Check sheet for the modelled part. Datum: model origin and axes. Units: mm. A direction names the side the tool comes from. Give positions to 0.01 mm unless a question says otherwise; leave off trailing zeros. Order: outer loops, then holes, each group sorted by start corner. A loop starts at its lowest first (then second) coordinate and runs counter-clockwise, first axis right, second up.
Autodesk Fusion 360 part; units mm, degrees
sketch "スケッチ1" plane through (0, 0, 0) normal (0, 0, 1) x (1, 0, 0)
  line L0 (0, 0) -> (20, 0)
  line L1 (20, 0) -> (20, 20)
  line L2 (20, 20) -> (0, 20)
  line L3 (0, 20) -> (0, 0)
  dimension "d1" = 20
  dimension "d2" = 20
extrude "押し出し1" add sketch "スケッチ1" along normal blind 21
sketch "スケッチ2" plane through (20, 0, 0) normal (1, 0, 0) x (0, 1, 0)
  line L0 (0, 0) -> (20, 0)
  line L1 (20, 0) -> (20, 21)
  line L2 (20, 21) -> (0, 21)
  line L3 (0, 21) -> (0, 0)
  circle A0 centre (5, 5) radius 1.15
  dimension "d5" = 2.3
  dimension "d8" = 5
  dimension "d11" = 5
extrude "押し出し2" cut sketch "スケッチ2" against normal blind 25 contours A0
sketch "スケッチ7" plane through (0, 0, 21) normal (0, 0, 1) x (-1, 0, 0)
  line L0 (0, -20) -> (0, 0)
  line L1 (0, 0) -> (-20, 0)
  line L2 (-20, 0) -> (-20, -20)
  line L3 (-20, -20) -> (0, -20)
  line L4 (-12.75, -17.75) -> (-20, -17.75)
  line L5 (-20, -17.75) -> (-20, -9.25)
  line L6 (-20, -9.25) -> (-12.75, -9.25)
  line L7 (-8.5, -13.5) -> (-20, -13.5)
  circle A0 centre (-12.85, -13.5) radius 1.6
  circle A1 centre (-16.85, -13.5) radius 1.6
  arc A2 (-12.75, -17.75) -> (-8.5, -13.5) centre (-12.75, -13.5) ccw
  arc A3 (-8.5, -13.5) -> (-12.75, -9.25) centre (-12.75, -13.5) ccw
  point P0 (-8.5, -17.75)
  point P1 (-8.5, -9.25)
  dimension "d16" = 8.5
  dimension "d17" = 11.5
  dimension "d18" = 3.2
  dimension "d19" = 3.2
  dimension "d20" = 4
  dimension "d21" = 4.35
  dimension "d22" = 4.25
  dimension "d23" = 4.25
  dimension "d24" = 4.25
extrude "押し出し4" cut sketch "スケッチ7" against normal blind 6.5 contours L2 L4 L5 L7 A0 A1 A2 | L2 L5 L6 L7 A0 A1 A3
extrude "押し出し5" cut 2 faces at (12.2215, 13.3267, 21) (16.1057, 13.3074, 21) along direction (0, 0, -1) blind 26
sketch "スケッチ11" plane through (20, 0, 0) normal (1, 0, 0) x (0, 1, 0)
  line L0 (17.75, 21) -> (17.75, 14.5)
  line L1 (17.75, 14.5) -> (9.25, 14.5)
  line L2 (9.25, 14.5) -> (9.25, 21)
  line L3 (9.25, 21) -> (0, 21)
  line L4 (0, 21) -> (0, 0)
  line L5 (0, 0) -> (20, 0)
  line L6 (20, 0) -> (20, 21)
  line L7 (20, 21) -> (17.75, 21)
  circle A0 centre (5, 5) radius 1.15
  line L8 (0, 10.5) -> (20, 10.5)
  line L9 (20, 10.5) -> (20, 0)
  line L10 (20, 0) -> (0, 0)
  line L11 (0, 0) -> (0, 10.5)
  dimension "d34" = 4
extrude "押し出し8" cut sketch "スケッチ11" against normal blind 32 contours L4 L5 L6 L8 L9 L10 L11
sketch "スケッチ12" plane through (0, 0, 21) normal (0, 0, 1) x (-1, 0, 0)
  line L0 (-12.75, -17.75) -> (-20, -17.75)
  line L1 (-20, -17.75) -> (-20, -20)
  line L2 (-20, -20) -> (0, -20)
  line L3 (0, -20) -> (0, 0)
  line L4 (0, 0) -> (-20, 0)
  line L5 (-20, 0) -> (-20, -9.25)
  line L6 (-20, -9.25) -> (-12.75, -9.25)
  arc A0 (-12.75, -17.75) -> (-12.75, -9.25) centre (-12.75, -13.5) ccw
  line L7 (-2.9, -12.6) -> (-6.1, -12.6)
  line L8 (-6.1, -12.6) -> (-6.1, -7.4)
  line L9 (-6.1, -7.4) -> (-2.9, -7.4)
  line L10 (-2.9, -7.4) -> (-2.9, -12.6)
  line L11 (-12.6, -2.9) -> (-7.4, -2.9)
  line L12 (-7.4, -2.9) -> (-7.4, -6.1)
  line L13 (-7.4, -6.1) -> (-12.6, -6.1)
  line L14 (-12.6, -6.1) -> (-12.6, -2.9)
  dimension "d37" = 2.9
  dimension "d38" = 5.2
  dimension "d39" = 3.2
  dimension "d40" = 7.4
  dimension "d41" = 3.2
  dimension "d42" = 5.2
  dimension "d43" = 2.9
  dimension "d44" = 7.4
extrude "押し出し9" cut sketch "スケッチ12" against normal blind 22 contours L7 L8 L9 L10 | L11 L12 L13 L14
equation "d40 = 10 mm - 2.6 mm"
1) Draft check along X on faces 4 (the face through (5, 7.4, 16)), 5 (the face through (10, 6.1, 16)), 6 (the face through (16, 17.75, 18)), 7 (the face through (20, 8, 15)). Enter one of: +X half, -X half, draft (parallel to the pull), parting line (faces both ways), or undercut.
Recorded:
face 4: undercut
face 5: undercut
face 6: draft
face 7: +X half
2) Depth check by flat-ended pin: pin 1 Ø1 at (x, y) = (17.5, 11) entering from +Z. Enter the tip coordinate at first touch or a pass-through.
Recorded:
pin 1: stops at z = 14.5
3) Section check D-D, the plane y = 13.5. Record the cut outline in (x, z), then the cut area to 3 significant figures.
Recorded:
outline: (0, 10.5) - (11.25, 10.5) - (11.25, 14.5) - (8.5, 14.5) - (8.5, 21) - (0, 21) - close; (14.45, 10.5) - (15.25, 10.5) - (15.25, 14.5) - (14.45, 14.5) - close; (18.45, 10.5) - (20, 10.5) - (20, 14.5) - (18.45, 14.5) - close
area: 110 mm2
4) Section check A-A, the plane x = 16.85. Record the cut outline in (y, z), then the cut area to 3 significant figures.
Recorded:
outline: (0, 10.5) - (11.9, 10.5) - (11.9, 14.5) - (9.25, 14.5) - (9.25, 21) - (0, 21) - close; (15.1, 10.5) - (20, 10.5) - (20, 21) - (17.75, 21) - (17.75, 14.5) - (15.1, 14.5) - close
area: 142 mm2
5) Set-up check for faces 1 (the face through (10, 10, 21)), 2 (the face through (8.5, 13.6, 17.8)), 3 (the face through (4, 12.6, 16)): record each of +Z, -Z, +X, -X, +Y, -Y from which the full face is reachable in a straight line by a thin tool's end or side.
Recorded:
face 1: +Z, +X, -X, +Y, -Y
face 2: +Z, +X
face 3: +Z, -Z
6) Section check C-C, the plane z = 19.5. Record the cut outline in (x, y), then the cut area to 3 significant figures.
Recorded:
outline: (0, 0) - (20, 0) - (20, 9.25) - (12.75, 9.25) arc R4.25 cw to (12.75, 17.75) - (20, 17.75) - (20, 20) - (0, 20) - close; hole (2.9, 7.4) - (6.1, 7.4) - (6.1, 12.6) - (2.9, 12.6) - close; hole (7.4, 2.9) - (12.6, 2.9) - (12.6, 6.1) - (7.4, 6.1) - close
area: 277 mm2
7) Section check B-B, the plane y = 5.25. Record the cut outline in (x, z).
Recorded:
outline: (0, 10.5) - (7.4, 10.5) - (7.4, 21) - (0, 21) - close; (12.6, 10.5) - (20, 10.5) - (20, 21) - (12.6, 21) - close
8) Material ranges on L1, parallel to X at y = 13.5, z = 11.45; L2, parallel to Y at x = 12.85, z = 13.5; L3, parallel to Y at x = 3.5, z = 14.25, recorded low to high.
Recorded:
L1: x = 0 to 11.25, 14.45 to 15.25, 18.45 to 20
L2: y = 0 to 11.9, 15.1 to 20
L3: y = 0 to 7.4, 12.6 to 20
